Here's how the part is built. I have some questions about the finished solid (model axes, mm). Face numbers are marked on the shaded views. A direction names the side the tool comes from. Round coordinates to 2 decimals unless told otherwise and drop trailing zeros. Order: outer loops, then holes, each group sorted by start corner. A loop starts at its lowest first (then second) coordinate and runs counter-clockwise, first axis right, second up.
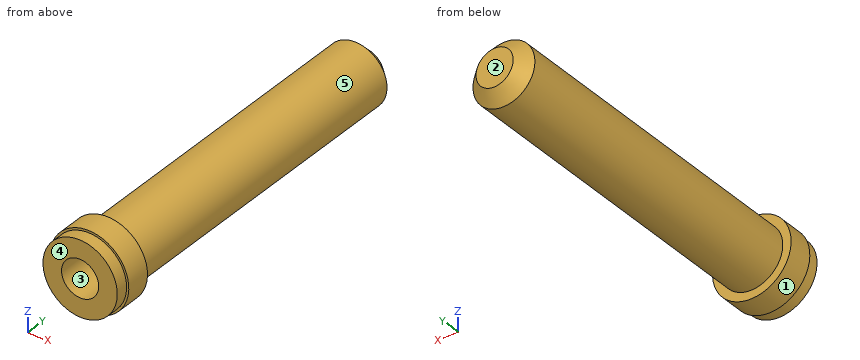
```python
from build123d import *

# Parameters (mm, degrees)
F3_SIZE2 = 2
F3_SIZE  = 2


# Not quite as in the source:
# - a feature names something its author has since deleted; it is built from what else it names


with BuildPart() as f1:
    # F0 (on Right) → F1 (revolve)
    with BuildSketch(Plane.YZ):
        Polygon((-7.8531129844, -6), (-5.8531129844, -6), (-5.8531129844, -6.35), (-1.8531129844, -6.35), (-1.8531129844, -5), (45.1962463558, -5), (53.1468870156, -5), (53.1468870156, 0), (7.1468870156, 0), (5, -3), (-7.8531129844, -3), (-7.8531129844, -5.5), align=None)
    revolve(axis=Axis((0, 30.1468870156, 0), (0, -1, 0)))

    # F3
    f3_edges = [f1.edges().sort_by_distance(p)[0] for p in [
        (0, 53.146887, 5),
    ]]
    chamfer(f3_edges, length=F3_SIZE, length2=F3_SIZE2)


solid = f1.part
```
1) I need wall thicknesses on line 1 (X direction, y = 1, z = 0); line 2 (X direction, y = -5, z = 0); line 3 (X direction, y = 13.5, z = -4). Which ranges of each line are inside material? Lowest first, please.
2) If we section it at A-A (y = -3): Write out the boundary of the cut face in (x, z).
3) If we section it at B-B (y = 32.5): Write out the boundary of the cut face in (x, z).
4) We'd pull the mould along X, two halves only. Please class the marked faces 1, 2 and 3: +X half, -X half, draft (parallel to the pull), parting line (faces both ways), or undercut.
5) For the marked faces 4 and 5, which set-ups out of +Z, -Z, +X, -X, +Y, -Y let a thin tool reach every point of the face, with its end or its side?
6) I'm going to push flat-ended pins straight in: pin 1 (2 mm diameter, centred on y = 42.5, z = 1, fed in from -X); pin 2 (1.5 mm diameter, centred on x = 1.5, z = -3, fed in from +Y); pin 3 (5 mm diameter, centred on x = -2.5, y = -0.5, fed in from -Z); pin 4 (1 mm diameter, centred on y = 18, z = -3.5, fed in from -X). Where does each tip first touch, or does it pass through?
Solutions:
1. line 1: x = -5 to -3, 3 to 5
1. line 2: x = -6.35 to -3, 3 to 6.35
1. line 3: x = -3 to 3
2. outline: circle Ø12.7 at (0, 0); hole circle Ø6 at (0, 0)
3. outline: circle Ø10 at (0, 0)
4. face 1: parting line
4. face 2: draft
4. face 3: undercut
5. face 4: +Z, -Z, +X, -X, -Y
5. face 5: +Y
6. pin 1: stops at x = -5
6. pin 2: stops at y = 53.15
6. pin 3: stops at z = -6.34
6. pin 4: stops at x = -4
